Autodesk Inventor part; units mm, degrees
ref_plane "Work Plane1" through (0, 16.25, -15) normal (0, 0, -1) x (-1, 0, 0)
ref_plane "YZ Plane" through (0, 0, 0) normal (1, 0, 0) x (0, 1, 0)
ref_plane "XZ Plane" through (0, 0, 0) normal (0, 1, 0) x (-1, 0, 0)
sketch "Sketch1" plane through (0, 0, 0) normal (1, 0, 0) x (0, 1, 0)
  line L0 (23.289, 22.5) -> (-23.289, 22.5)
  line L1 (-23.289, 22.5) -> (-23.289, -22.5)
  line L2 (-23.289, -22.5) -> (23.289, -22.5)
  line L3 (23.289, -22.5) -> (23.289, 22.5)
  line L4 (23.289, 22.5) -> (-23.289, -22.5) construction
  line L5 (-23.289, 22.5) -> (23.289, -22.5) construction
  point P0 (0, 0)
  dimension "d0" = 45
  dimension "d1" = 46.578
extrude "Extrusion1" add sketch "Sketch1" along normal blind 50
fillet "Fillet1" radius 0.01 2 edges at (50, 0, 22.5) (0, 0, 22.5)
sketch "Sketch2" plane through (0.01, -23.289, 22.5) normal (0, 0, 1) x (1, 0, 0)
  arc A0 (21.5019, 41.5691) -> (18.149, 39.3946) centre (19.8721, 40.41) ccw
  line L0 (24.1767, 29.1655) -> (18.149, 39.3946)
  circle A1 centre (19.7361, 40.6197) radius 0.65
  circle A2 centre (20.8243, 38.9417) radius 0.65
  line L1 (21.5019, 41.5691) -> (28.3834, 31.8938)
  circle A3 centre (21.9126, 37.2637) radius 0.65
  circle A4 centre (23.0009, 35.5857) radius 0.65
  circle A5 centre (24.0892, 33.9077) radius 0.65
  circle A6 centre (25.1774, 32.2297) radius 0.65
  circle A7 centre (29.8026, 25.0983) radius 0.65
  circle A8 centre (27.49, 28.664) radius 3.325
  line L2 (33.4781, 15.7589) -> (26.5966, 25.4342)
  arc A9 (33.4781, 15.7589) -> (36.831, 17.9334) centre (35.1079, 16.918) ccw
  line L3 (30.8033, 28.1625) -> (36.831, 17.9334)
  circle A10 centre (30.8908, 23.4203) radius 0.65
  circle A11 centre (31.9791, 21.7423) radius 0.65
  circle A12 centre (33.0674, 20.0643) radius 0.65
  circle A13 centre (34.1557, 18.3863) radius 0.65
  circle A14 centre (35.2439, 16.7083) radius 0.65
  line L4 (24.1767, 29.1655) -> (24.1978, 29.1297)
  line L5 (30.8033, 28.1625) -> (30.7822, 28.1983)
  line L6 (26.5966, 25.4342) -> (26.5725, 25.4681)
  line L7 (28.3834, 31.8938) -> (28.4075, 31.8599)
  point P0 (-0.01, 23.289)
extrude "Extrusion2" cut sketch "Sketch2" against normal blind 2.35 contours L1 L7 A8 L4 L0 A0 | A8 | A8 L5 L3 A9 L2 L6 | A1 | A2 | A3 | A4 | A5 | A6 | A7 | A10 | A11 | A12 | A13 | A14
sketch "Sketch3" plane through (0.01, -23.289, 22.5) normal (0, 0, 1) x (1, 0, 0)
  circle A0 centre (20.8243, 38.9417) radius 0.65
  circle A1 centre (19.7361, 40.6197) radius 0.65
  circle A2 centre (21.9126, 37.2637) radius 0.65
  circle A3 centre (23.0009, 35.5857) radius 0.65
  circle A4 centre (24.0892, 33.9077) radius 0.65
  circle A5 centre (25.1774, 32.2297) radius 0.65
  circle A6 centre (29.8026, 25.0983) radius 0.65
  circle A7 centre (30.8908, 23.4203) radius 0.65
  circle A8 centre (31.9791, 21.7423) radius 0.65
  circle A9 centre (33.0674, 20.0643) radius 0.65
  circle A10 centre (34.1557, 18.3863) radius 0.65
  circle A11 centre (35.2439, 16.7083) radius 0.65
  point P0 (-0.01, 23.289)
extrude "Extrusion3" cut sketch "Sketch3" against normal blind 10
sketch "Sketch4" plane through (50, 0, 0) normal (1, 0, 0) x (0, 0, -1)
  line L0 (30, 4) -> (30, -4)
  line L1 (30, -4) -> (15, -4)
  line L2 (15, -4) -> (15, 4)
  line L3 (15, 4) -> (30, 4)
  line L4 (62.5, 16.25) -> (-17.5, 16.25)
  line L5 (62.5, -16.25) -> (-17.5, -16.25)
  line L6 (-17.5, 16.25) -> (-17.5, -16.25)
  line L7 (62.5, 16.25) -> (62.5, -16.25)
  point P0 (0, 0)
extrude "Extrusion4" cut sketch "Sketch4" against normal through all contours L0 L1 L2 L3 | L7 L5 L6 L4
sketch "Sketch5" plane through (0, 23.289, -22.5) normal (0, 1, 0) x (1, 0, 0)
  line L0 (0, 0) -> (50, 0)
  line L1 (50, 0) -> (45, 0)
  line L2 (45, 0) -> (45, -48.3734)
  line L3 (45, -48.3734) -> (50, -48.3734)
  line L4 (50, -48.3734) -> (50, 0)
  point P0 (0, -22.5)
  point P1 (45, 0)
  dimension "d11" = 5
extrude "Extrusion5" cut sketch "Sketch5" against normal through all
sketch "Sketch6" plane through (0, 23.289, 22.49) normal (0, 1, 0) x (1, 0, 0)
  line L0 (45, 4.99) -> (45, 44.99)
  line L1 (45, 44.99) -> (37, 44.99)
  line L2 (37, 44.99) -> (37, -0.01)
  line L3 (37, -0.01) -> (45, -0.01)
  line L4 (45, -0.01) -> (45, 44.99)
  line L5 (0.01, -0.01) -> (45, -0.01)
  point P0 (0, 22.49)
  point P1 (45, 9.99)
  point P2 (41, -0.01)
  point P3 (45, 9.99)
  dimension "d14" = 0
  dimension "d15" = 8
extrude "Extrusion6" add sketch "Sketch6" against normal up to surface (39.539 mm away)
sketch "Sketch7" plane through (0, -23.289, -22.5) normal (0, 0, -1) x (-1, 0, 0)
  line L0 (-41, 21.289) -> (-44.4641, 21.289)
  arc A0 (-44.4641, 21.289) -> (-41, 19.289) centre (-41, 23.289) ccw
  line L1 (-41, 19.289) -> (-37, 19.289)
  line L2 (-37, 27.289) -> (-37, 19.289)
  line L3 (-37, 27.289) -> (-41, 27.289)
  arc A1 (-41, 27.289) -> (-44.4641, 25.289) centre (-41, 23.289) ccw
  line L4 (-44.4641, 25.289) -> (-41, 25.289)
  arc A2 (-41, 21.289) -> (-41, 25.289) centre (-41, 23.289) ccw
  arc A3 (-44.4641, 25.289) -> (-44.4641, 21.289) centre (-41, 23.289) ccw
  arc A4 (-41, 25.289) -> (-41, 21.289) centre (-41, 23.289) ccw
  arc A5 (-41, 25.289) -> (-41, 21.289) centre (-41, 23.289) ccw
  line L5 (-44.4641, 25.289) -> (-41, 25.289)
  arc A6 (-44.4641, 25.289) -> (-44.4641, 21.289) centre (-41, 23.289) ccw
  line L6 (-41, 21.289) -> (-44.4641, 21.289)
  point P0 (0, 23.289)
sketch "Sketch8" plane through (0, 23.289, 22.49) normal (0, 1, 0) x (1, 0, 0)
  line L0 (0.01, -0.01) -> (45, -0.01)
  line L1 (45, -0.01) -> (40, -0.01)
  line L2 (40, -0.01) -> (40, 55.178)
  line L3 (40, 55.178) -> (45, 55.178)
  line L4 (45, 55.178) -> (45, -0.01)
  point P0 (0, 22.49)
  point P1 (40, -0.01)
  dimension "d18" = 5
extrude "Extrusion7" cut sketch "Sketch8" against normal through all
extrude "Extrusion8" cut sketch "Sketch7" against normal blind 7.5
ref_plane "Work Plane1" through (0, 16.25, -15) normal (0, 0, -1) x (-1, 0, 0)
sketch "Sketch9" plane through (0, 16.25, -15) normal (0, 0, -1) x (-1, 0, 0)
  arc A0 (-41, -12.25) -> (-44.4641, -14.25) centre (-41, -16.25) ccw
  line L0 (-37, -12.25) -> (-41, -12.25)
  line L1 (-37, -12.25) -> (-37, -20.25)
  arc A1 (-41, -18.25) -> (-41, -14.25) centre (-41, -16.25) ccw
  arc A2 (-41, -14.25) -> (-41, -18.25) centre (-41, -16.25) ccw
  line L2 (-41, -18.25) -> (-44.4641, -18.25)
  line L3 (-44.4641, -14.25) -> (-41, -14.25)
  arc A3 (-44.4641, -14.25) -> (-44.4641, -18.25) centre (-41, -16.25) ccw
  arc A4 (-44.4641, -18.25) -> (-41, -20.25) centre (-41, -16.25) ccw
  line L4 (-37, -20.25) -> (-40, -20.25)
  line L5 (-41, -20.25) -> (-37, -20.25)
  line L6 (-40, -12.25) -> (-40, -20.25)
  line L7 (-40, -39.539) -> (-40, 7.039)
  line L8 (-39, -12.25) -> (-39, -20.25)
  point P0 (0, -16.25)
  point P1 (-39, -20.25)
  point P2 (-39, -16.25)
extrude "Extrusion9" cut sketch "Sketch9" against normal blind 5 contours L0 L6 A1 L3 A0 | L3 A2 L2 A3 | L0 L8 A1 L6 | A1 L6 A2 | L2 A1 L6 L5 A4 | A1 L6 | L8 L4 L6 A1
extrude "Extrusion10" add sketch "Sketch9" against normal blind 5 contours L0 L6 A1 L3 A0 | L3 A2 L2 A3 | L0 L8 A1 L6 | L2 A1 L6 L5 A4 | L8 L4 L6 A1
extrude "Extrusion11" cut sketch "Sketch9" against normal blind 10 contours A1 L6 A2 | A1 L6
sketch "Sketch10" plane through (0, 23.289, 22.49) normal (0, 1, 0) x (1, 0, 0)
  line L0 (0, -0.01) -> (13, -0.01)
  line L1 (13, -0.01) -> (13, 49.0312)
  line L2 (13, 49.0312) -> (0, 49.0312)
  line L3 (0, 49.0312) -> (0, -0.01)
  line L4 (0, 44.99) -> (0, 0)
  line L5 (0.01, -0.01) -> (40, -0.01)
  point P0 (0, 22.49)
  dimension "d30" = 0
  dimension "d31" = 13
  dimension "d32" = 0
extrude "Extrusion12" cut sketch "Sketch10" against normal through all
sketch "Sketch11" plane through (40, 4, -22.5) normal (0, 0, -1) x (-1, 0, 0)
  line L0 (27, 12.25) -> (27, 19.289)
  line L1 (27, 19.289) -> (0, 19.289)
  line L2 (0, 19.289) -> (0, 0)
  line L3 (0, 0) -> (3, 0)
  line L4 (3, 12.25) -> (3, 0)
  line L5 (3, 12.25) -> (27, 12.25)
  line L6 (27, -27.289) -> (27, -20.25)
  line L7 (27, -20.25) -> (3, -20.25)
  line L8 (3, -8) -> (3, -20.25)
  line L9 (3, -8) -> (0, -8)
  line L10 (0, -8) -> (0, -27.289)
  line L11 (27, -27.289) -> (0, -27.289)
  point P0 (40, -4)
extrude "Extrusion13" add sketch "Sketch11" along normal blind 40
fillet "Fillet2" radius 3 12 edges at (26.5, 23.289, -62.5) (40, 13.6445, -62.5) (13, 23.289, -20) (13, -23.289, -20) (26.5, -23.289, -62.5) (40, -13.6445, -62.5) (13, 0, 22.5) (40, 0, 22.5) (26.5, -23.289, 22.5) (26.5, 23.289, 22.5) (40, 23.289, -20) (40, -23.289, -20)
properties part number "New End effector"
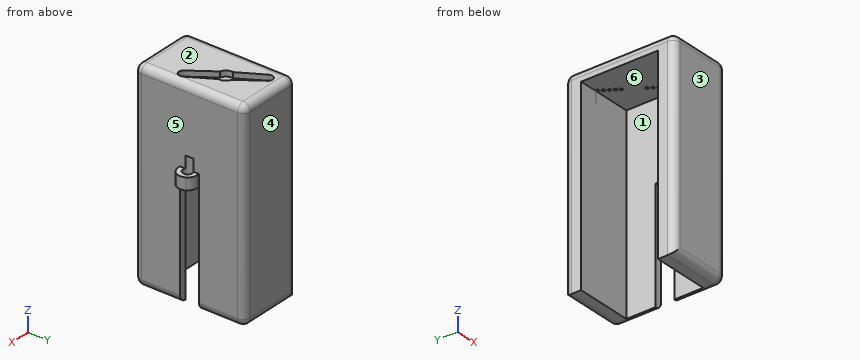
Check sheet for the modelled part. Datum: model origin and axes. Units: mm. Face numbers are marked on the shaded views. A direction names the side the tool comes from. Round coordinates to 2 decimals unless told otherwise and drop trailing zeros. Write each loop counter-clockwise with the first axis right and the second up, starting at its lowest first coordinate (ties: lowest second). Pieces come first, ordered by that corner, then holes. Notation, with made-up numbers: (76, 83.25) - (113, 83.25) arc R20 cw to (113, 103.25) - close; hole circle Ø6 at (-6.75, -30). An arc over 180 degrees is marked (long way). Return JSON: item names as keys, results as strings.
Q1. Depth check by flat-ended pin: P1, Ø1.5, axis at y = 18.5, z = 2.5, coming from the +X side; P2, Ø2, axis at x = 26.5, y = 6.5, coming from the +Z side; P3, Ø1, axis at x = 32, y = -2, coming from the -Z side; P4, Ø1, axis at x = 24.5, y = 4.5, coming from the +Z side. Enter the tip coordinate at first touch or a pass-through.
Returned:
{"P1": "stops at x = 40", "P2": "stops at z = 20.15", "P3": "stops at z = 17.5", "P4": "stops at z = 22.5"}
Q2. Access from +Z, -Z, +X, -X, +Y, -Y to the whole of each face (thin tool, end or side, straight path). Record for the marked faces 1 and 2.
Returned:
{"face 1": "-Z, -X", "face 2": "+Z, +X, -X, +Y, -Y"}
Q3. Draft check along Y on the marked faces 3, 4, 5 and 6. Enter one of: released by +Y, released by -Y, zero draft, split by the parting line, or undercut.
Returned:
{"face 3": "released by -Y", "face 4": "released by +Y", "face 5": "zero draft", "face 6": "undercut"}
Q4. Scan lines: L1, parallel to Y at x = 21.5, z = -41; L2, parallel to Z at x = 34, y = 2; L3, parallel to X at y = -4.5, z = -49. Record each from-to range of solid material in increasing order. Write a range as from..to.
Returned:
{"L1": "y = -23.29..-16.25, 16.25..23.29", "L2": "z = 17.5..22.5", "L3": "x = 37..40"}
Q5. Cross-section at A-A (z = -31). Record the boundary of the cut face in (x, y), then the cut area to 3 significant figures.
Returned:
{"outline": "(13, -20.29) arc R3 ccw to (16, -23.29) - (37, -23.29) arc R3 ccw to (40, -20.29) - (40, -4) - (37, -4) - (37, -16.25) - (13, -16.25) - close; (13, 16.25) - (37, 16.25) - (37, 4) - (40, 4) - (40, 20.29) arc R3 ccw to (37, 23.29) - (16, 23.29) arc R3 ccw to (13, 20.29) - close", "area": "446 mm²"}
